from build123d import *

# Parameters (mm, degrees)
F0_W     = 150
F0_H     = 140
F1_DEPTH = 2
F2_R     = 2.5
F3_DEPTH = 5
F4_R     = 50
F4_R_2   = 49.75
F5_DEPTH = 1
F6_R     = 10
F6_R_2   = 9.75
F7_DEPTH = 1


with BuildPart() as f1:
    # F0 (on Top) → F1 (new body)
    with BuildSketch(Plane.XY):
        Rectangle(F0_W, F0_H)
    extrude(amount=F1_DEPTH)

    # F2 (on face) → F3 (cut)
    with BuildSketch(Plane.XY.offset(2)):
        Polygon((-75, 70), (-75, 41.5), (-46.5, 70), align=None)
        with Locations((-64, 57.6)):
            Circle(F2_R, mode=Mode.SUBTRACT)
        Polygon((-46.5, -70), (-75, -41.5), (-75, -70), align=None)
        with Locations((-64, -57.6)):
            Circle(F2_R, mode=Mode.SUBTRACT)
        with BuildLine():
            Line((-67.1845650673, -6.35), (-67.1845650673, 6.35))
            ThreePointArc((-67.1845650673, 6.35), (-67.9167981143, 8.117766953), (-69.6845650673, 8.85))
            Line((-69.6845650673, 8.85), (-75, 8.85))
            Line((-75, 8.85), (-75, -8.85))
            Line((-75, -8.85), (-69.6845650673, -8.85))
            ThreePointArc((-69.6845650673, -8.85), (-67.9167981143, -8.117766953), (-67.1845650673, -6.35))
        make_face()
        with BuildLine():
            Line((-21.499911428, -66.5210440509), (-22.940942165, -70))
            Line((-22.940942165, -70), (-14.8778247705, -70))
            Line((-14.8778247705, -70), (-16.500088572, -66.5210440509))
            ThreePointArc((-16.500088572, -66.5210440509), (-19, -64), (-21.499911428, -66.5210440509))
        make_face()
        with BuildLine():
            Line((-14.8778247705, 70), (-22.940942165, 70))
            Line((-22.940942165, 70), (-21.499911428, 66.5210440509))
            ThreePointArc((-21.499911428, 66.5210440509), (-19, 64), (-16.500088572, 66.5210440509))
            Line((-16.500088572, 66.5210440509), (-14.8778247705, 70))
        make_face()
        with Locations((-64, 57.6)):
            Circle(F2_R)
        with Locations((-64, -57.6)):
            Circle(F2_R)
    extrude(amount=-F3_DEPTH, mode=Mode.SUBTRACT)

    # F4 (on face) → F5 (join)
    with BuildSketch(Plane.XY.offset(2)):
        with Locations((-3.16328, 0)):
            Circle(F4_R)
        with Locations((-3.16328, 0)):
            Circle(F4_R_2, mode=Mode.SUBTRACT)
    extrude(amount=F5_DEPTH)

    # F6 (on face) → F7 (join)
    with BuildSketch(Plane.XY.offset(2)):
        with Locations((-3.16328, 0)):
            Circle(F6_R)
        with Locations((-3.16328, 0)):
            Circle(F6_R_2, mode=Mode.SUBTRACT)
    extrude(amount=F7_DEPTH)


solid = f1.part
Source: CAD feature listing. Evaluate the final solid. Frame: model axes, mm. A direction names the side the tool comes from. Round coordinates to 2 decimals unless told otherwise and drop trailing zeros. Loops run counter-clockwise (first coordinate to the right, second up) from the corner with the lowest first, then second, coordinate; pieces in that order, holes last. Notation, with made-up numbers: M 75.5,-9 L 133.5,-9 A11 ccw 133.5,2 Z; hole C 17.25,77.5 d5. An arc over 180 degrees is marked long. Return JSON: item names as keys, results as strings. Group by question number.
1. Section query C-C on y = -61. Output: boundary loops of the cut face in (x, z), and give its area (3 significant figures).
2. Mould query, pull axis Y, two halves, no side actions, for faces 3 (the face through (-60.9, 55.6, 1)), 4 (the face through (-3.9, -10.4, 2)), 5 (the face through (-3, 0, 2)), 6 (the face through (44.528, 15.019, 2.493)). Classes: released by +Y, released by -Y, zero draft, split by the parting line, or undercut.
3. Section query B-B on x = 34. Output: boundary loops of the cut face in (y, z), and give its area (3 significant figures).
4. Section query A-A on y = 0. Output: boundary loops of the cut face in (x, z), and give its area (3 significant figures).
5. Reachability of faces 1 (the face through (-5.331, -9.762, 2.493)), 2 (the face through (-1, 1, 0)) from +Z, -Z, +X, -X, +Y, -Y: full face, straight path, thin tool, end or side. Return the list, or none.
6. Pin query (flat end, axial travel): pin 1 (6 mm diameter, centred on x = -4.5, y = 0, fed in from +Z); pin 2 (0.6 mm diameter, centred on x = -73, z = 1, fed in from -Y). Return the tip coordinate at first contact, or that it passes through.
7. Material intervals for line 1 along Z through (x, y) = (-35, -9); line 2 along Y through (x, z) = (-50, 0.75); line 3 along X through (y, z) = (11, 2.35), sorted ascending. Write a range as from..to.
8. Section query D-D on x = -19. Output: boundary loops of the cut face in (y, z), and give its area (3 significant figures).
Checks:
{
 "1": {"outline": "M -55.5,0 L 75,0 L 75,2 L -55.5,2 Z", "area": "261 mm²"},
 "2": {"face 3": "released by +Y", "face 4": "undercut", "face 5": "undercut", "face 6": "split by the parting line"},
 "3": {"outline": "M -70,0 L 70,0 L 70,2 L 33.45,2 L 33.45,3 L 33.07,3 L 33.07,2 L -33.07,2 L -33.07,3 L -33.45,3 L -33.45,2 L -70,2 Z", "area": "281 mm²"},
 "4": {"outline": "M -67.18,0 L 75,0 L 75,2 L 46.84,2 L 46.84,3 L 46.59,3 L 46.59,2 L 6.84,2 L 6.84,3 L 6.59,3 L 6.59,2 L -12.91,2 L -12.91,3 L -13.16,3 L -13.16,2 L -52.91,2 L -52.91,3 L -53.16,3 L -53.16,2 L -67.18,2 Z", "area": "285 mm²"},
 "5": {"face 1": "+Z", "face 2": "-Z, +X, -X, +Y, -Y"},
 "6": {"pin 1": "stops at z = 2", "pin 2": "stops at y = -43.8"},
 "7": {"line 1": "z = 0..2", "line 2": "y = -66.5..66.5", "line 3": "x = -51.94..-51.68, 45.36..45.61"},
 "8": {"outline": "M -64,0 L 64,0 L 64,2 L 47.43,2 L 47.43,3 L 47.16,3 L 47.16,2 L -47.16,2 L -47.16,3 L -47.43,3 L -47.43,2 L -64,2 Z", "area": "257 mm²"}
}
